Model file for the job. Use its own axes, mm. A direction names the side the tool comes from. Coordinates: 2 decimals unless noted, no trailing zeros. Write each loop counter-clockwise with the first axis right and the second up, starting at its lowest first coordinate (ties: lowest second). Pieces come first, ordered by that corner, then holes. Notation, with made-up numbers: M -10.5,24 L 45.5,24 A30 cw 45.5,54 Z; hole C -28,86.5 d3. An arc over 180 degrees is marked long. Put each result on its own line as item: value. Start each with the question number.
Q1. Cut at B-B (y = 3). Write the cut outline in (x, z), then the cut area to 3 significant figures.
Q2. Cut at C-C (z = -20). Write the cut outline in (x, y), then the cut area to 3 significant figures.
Q3. Drop flat-ended pins along their axis: pin 1 (5 mm diameter, centred on x = 2, z = -8, fed in from -Y); pin 2 (0.9 mm diameter, centred on x = -3.5, z = -24, fed in from +Y); pin 3 (4 mm diameter, centred on x = -3.5, y = 8, fed in from +Z); pin 4 (3 mm diameter, centred on x = 0.5, y = 5.5, fed in from +Z). Give the stop position or say it passes through.
Q4. Drill centre lines: line 1 along Y through (x, z) = (2.25, -16.5); line 2 along Z through (x, y) = (0, 10.05); line 3 along X through (y, z) = (9.25, -2). Where is each one in solid material? Low to high.
Q5. Cut at D-D (y = 5.5). Write the cut outline in (x, z), then the cut area to 3 significant figures.
Q6. Which spindle directions (+Z, -Z, +X, -X, +Y, -Y) get a long thin tool onto all of the face, cutting with end or side? Do faces 4 (the flat face through (-3, 7, -27)), 5 (the cylindrical face through (3.52, -5.05, -1.43)), 6 (the flat face through (-2, -7, -21)), 7 (the flat face through (-4, 5, -21)). Say none if no direction does.
Q7. Pull direction X, two halves, no side cores. Call faces 1 (the flat face through (5, -2, -10)), 2 (the flat face through (-4, -5, -21)), 3 (the flat face through (-2, 7, -21)): pulls with the +X half, pulls with the -X half, needs draft (parallel to the pull), parting line crosses it, or undercut.
Q8. Cut at A-A (x = 0). Write the cut outline in (y, z), then the cut area to 3 significant figures.
Autodesk Inventor part; units mm, degrees
ref_plane "YZ Plane" through (0, 0, 0) normal (1, 0, 0) x (0, 1, 0)
ref_plane "XZ Plane" through (0, 0, 0) normal (0, 1, 0) x (-1, 0, 0)
ref_plane "XY Plane" through (0, 0, 0) normal (0, 0, 1) x (1, 0, 0)
sketch "Sketch1" plane through (0, 0, 0) normal (0, 1, 0) x (-1, 0, 0)
  circle A0 centre (0, 0) radius 5
  circle A1 centre (0, 0) radius 2.5
extrude "Extrusion1" add sketch "Sketch1" along normal mid plane 21
sketch "Sketch2" plane through (0, 0, 0) normal (0, 1, 0) x (-1, 0, 0)
  circle A0 centre (0, 0) radius 5 construction
  line L0 (5, 0) -> (5, -27) construction
  line L1 (5, 0) -> (-5, 0)
  line L2 (-5, 0) -> (-5, -27)
  line L3 (-5, -27) -> (5, -27)
  line L4 (5, -27) -> (5, 0)
  dimension "d4" = 27
extrude "Extrusion2" add sketch "Sketch2" along normal mid plane 18
sketch "Sketch3" plane through (0, 9, 0) normal (0, 1, 0) x (1, 0, 0)
  circle A0 centre (0, 0) radius 2.5
extrude "Extrusion3" cut sketch "Sketch3" against normal blind 18
sketch "Sketch4" plane through (0, 9, 0) normal (0, 1, 0) x (1, 0, 0)
  line L0 (5, 0) -> (5, 27)
  arc A0 (-2, 15) -> (2, 15) centre (0, 15) ccw
  line L1 (2, 27) -> (2, 15)
  line L2 (-2, 27) -> (-2, 15)
  line L3 (2, 27) -> (-2, 27)
  line L4 (5, 27) -> (-5, 27)
  point P0 (0, 0)
extrude "Extrusion4" cut sketch "Sketch4" against normal through all
sketch "Sketch5" plane through (-5, -9, 0) normal (-1, 0, 0) x (0, 0, 1)
  line L0 (-27, 18) -> (-27, 14) construction
  line L1 (-27, 14) -> (-27, 4)
  line L2 (-27, 0) -> (-27, 18)
  line L3 (-27, 9) -> (-10, 9) construction
  arc A0 (-15, 4) -> (-15, 14) centre (-15, 9) ccw
  line L4 (-27, 14) -> (-15, 14)
  line L5 (-27, 4) -> (-15, 4)
  point P0 (0, 9)
  dimension "d16" = 10
  dimension "d17" = 17
extrude "Extrusion5" cut sketch "Sketch5" against normal through all
sketch "Sketch7" plane through (5, -9, 0) normal (1, 0, 0) x (0, 0, -1)
  line L0 (-5, -1.5) -> (5, -1.5) construction
  line L1 (0, -1.5) -> (0, 3.5) construction
  line L2 (0, 0) -> (0, 18) construction
  line L3 (5, 19.5) -> (-5, 19.5) construction
  line L4 (0, 19.5) -> (0, 14.5) construction
  circle A0 centre (0, 3.5) radius 1.5
  circle A1 centre (0, 14.5) radius 1.5
  point P0 (0, 9)
  dimension "d28" = 5
  dimension "d29" = 5
  dimension "d30" = 3
  dimension "d31" = 3
extrude "Extrusion7" cut sketch "Sketch7" against normal up to surface
properties part number "Forcella"
Computed values:
1. outline: M -5,-11 L 5,-11 L 5,0 A5 ccw -5,0 Z; hole C 0,0 d5
1. area: 130 mm2
2. outline: M -5,-9 L -2,-9 L -2,-5 L -5,-5 Z; M -5,5 L -2,5 L -2,9 L -5,9 Z; M 2,-9 L 5,-9 L 5,-5 L 2,-5 Z; M 2,5 L 5,5 L 5,9 L 2,9 Z
2. area: 48.0 mm2
3. pin 1: y = -9
3. pin 2: y = 9
3. pin 3: z = 4.77
3. pin 4: z = 5
4. line 1: -9 to -5, 5 to 9
4. line 2: -5 to -2.5, 2.5 to 5
4. line 3: -4.58 to -1.5, 1.5 to 4.58
5. outline: M -5,-27 L -2,-27 L -2,-15 A2 cw 2,-15 L 2,-27 L 5,-27 L 5,-1.5 L 2,-1.5 A2.5 cw long 2,1.5 L 4.77,1.5 A5 ccw -5,0 Z
5. area: 227 mm2
6. face 4: -Z, +X, -X, +Y, -Y
6. face 5: +X
6. face 6: -Z, +Y, -Y
6. face 7: -Z, +X, -X
7. face 1: pulls with the +X half
7. face 2: needs draft
7. face 3: undercut
8. outline: M -10.5,-5 L -9,-5 L -9,-13 L -4.58,-13 A5 cw 4.58,-13 L 9,-13 L 9,-5 L 10.5,-5 L 10.5,-2.5 L -10.5,-2.5 Z; M -10.5,2.5 L 10.5,2.5 L 10.5,5 L -10.5,5 Z
8. area: 229 mm2
